```python
from build123d import *

# Parameters (mm, degrees)
BOSS_EXTRUDE1_DEPTH      = 1
SKETCH2_W                = 9
SKETCH2_H                = 4
BOSS_EXTRUDE2_DEPTH      = 1.5
BOSS_EXTRUDE5_DEPTH      = 8
BOSS_EXTRUDE5_DEPTH_BACK = 8


with BuildPart() as part:
    # Sketch1 → Boss-Extrude1 (new body)
    with BuildSketch(Plane.XY):
        Polygon((-63, -10), (-70, -10), (-70, 10), (-63, 10), (-63, 30.8), (-110.8, 30.8), (-110.8, -30.8), (-63, -30.8), align=None)
    extrude(amount=-BOSS_EXTRUDE1_DEPTH)

    # Sketch2 → Boss-Extrude2 (add)
    with BuildSketch(Plane(origin=(0, 0, -1), x_dir=(-1, 0, 0), z_dir=(0, 0, -1))):
        with Locations((110.8, -10)):
            Rectangle(SKETCH2_W, SKETCH2_H)
        with Locations((110.8, 10)):
            Rectangle(SKETCH2_W, SKETCH2_H)
    extrude(amount=BOSS_EXTRUDE2_DEPTH)

    # Sketch4 → Boss-Extrude5 (add, two sides: drawn at the far end of the back side and taken through both)
    with BuildSketch(Plane(origin=(0, 0, 0), x_dir=(1, 0, 0), z_dir=(0, 1, 0)).offset(-BOSS_EXTRUDE5_DEPTH_BACK)):
        with BuildLine():
            Line((-63.746646239, 13.303022537), (-63.062370045, 2))
            Line((-63.062370045, 2), (-64.5, 2))
            Line((-64.5, 2), (-64.5, -0.2))
            Line((-64.5, -0.2), (-63.5, -0.2))
            Line((-63.5, -0.2), (-63.5, 1))
            Line((-63.5, 1), (-62, 1))
            Line((-62, 1), (-62.790668189, 14.060428588))
            ThreePointArc((-62.790668189, 14.060428588), (-63.7786518, 14.999948092), (-64.785574648, 14.080755571))
            Line((-64.785574648, 14.080755571), (-65.688532626, 2.935903953))
            ThreePointArc((-65.688532626, 2.935903953), (-66.359873651, 1.557863976), (-67.787627389, 1))
            Line((-67.787627389, 1), (-70, 1))
            Line((-70, 1), (-70, 0))
            Line((-70, 0), (-67.787627389, 0))
            ThreePointArc((-67.787627389, 0), (-65.681919218, 0.822760048), (-64.691798691, 2.855148382))
            Line((-64.691798691, 2.855148382), (-63.845228573, 13.304027036))
            ThreePointArc((-63.845228573, 13.304027036), (-63.795469446, 13.349450792), (-63.746646239, 13.303022537))
        make_face()
    extrude(amount=BOSS_EXTRUDE5_DEPTH + BOSS_EXTRUDE5_DEPTH_BACK)


solid = part.part
```
Read the model definition and answer for the solid it produces. Units are mm, in the model's axes. A direction names the side the tool comes from. Round coordinates to 2 decimals unless told otherwise and drop trailing zeros. Write each loop counter-clockwise with the first axis right and the second up, starting at its lowest first coordinate (ties: lowest second). Pieces come first, ordered by that corner, then holes. Notation, with made-up numbers: (-32.5, -20) - (7.5, -20) arc R9 cw to (7.5, -12) - close; hole circle Ø1 at (3.25, 77). An arc over 180 degrees is marked (long way). One line per item, written item: value.
Q1. Find section A-A (y = 2). Determine the outline of the cut face in (x, z), and give its area (3 significant figures).
The answers:
outline: (-110.8, -1) - (-67.79, -1) arc R2.11 cw to (-65.69, -2.94) - (-64.79, -14.08) arc R1 ccw to (-62.79, -14.06) - (-62, -1) - (-63.5, -1) - (-63.5, 0.2) - (-64.5, 0.2) - (-64.5, -2) - (-63.06, -2) - (-63.75, -13.3) arc R0.05 cw to (-63.85, -13.3) - (-64.69, -2.86) arc R3.11 ccw to (-67.79, 0) - (-110.8, 0) - close
area: 75.3 mm2
Q2. Find section D-D (y = -21). Determine the outline of the cut face in (x, z).
The answers:
outline: (-110.8, -1) - (-63, -1) - (-63, 0) - (-110.8, 0) - close
Q3. Find section C-C (x = -103). Determine the outline of the cut face in (y, z), and give its area (3 significant figures).
The answers:
outline: (-30.8, -1) - (30.8, -1) - (30.8, 0) - (-30.8, 0) - close
area: 61.6 mm2
Q4. Straight lines are drawn through the part: line 1 (Y direction, x = -109, z = -1.5); line 2 (Z direction, x = -87.5, y = -19); line 3 (Z direction, x = -112, y = -9). For each, find the intervals that lie inside material, in ascending order. Write a range as from..to.
The answers:
line 1: y = -12..-8, 8..12
line 2: z = -1..0
line 3: z = -2.5..-1
Q5. Which of the six approach directions +Z, -Z, +X, -X, +Y, -Y give full straight-line access (tool end or side, diameter ignored) to faces 5 (the flat face through (-65, -8, -6)), 6 (the flat face through (-113, 10, -1)), 7 (the flat face through (-115.3, 10, -2)), 8 (the flat face through (-106.3, -10, -2)), 9 (the flat face through (-64.274, -0.112, -8.006))?
The answers:
face 5: +Z, -Z, +X
face 6: +Z, -X, +Y, -Y
face 7: +Z, -Z, -X, +Y, -Y
face 8: -Z, +X, +Y, -Y
face 9: +Y, -Y
Q6. Find section B-B (z = -12). Determine the outline of the cut face in (x, y).
The answers:
outline: (-64.95, -8) - (-63.95, -8) - (-63.95, 8) - (-64.95, 8) - close; (-63.67, -8) - (-62.67, -8) - (-62.67, 8) - (-63.67, 8) - close
Q7. For a pull along Y with two mould halves and no side action, classify faces 1 (the flat face through (-111, 12, -2)), 2 (the flat face through (-64, 0, -2)), 3 (the flat face through (-111, 8, -2)), 4 (the flat face through (-111, -12, -2)) as pulls with the +Y half, pulls with the -Y half, needs draft (parallel to the pull), parting line crosses it, or undercut.
The answers:
face 1: pulls with the +Y half
face 2: needs draft
face 3: undercut
face 4: pulls with the -Y half
Q8. Each of these flat-tipped pins is pushed along its axis until it touches: P1, Ø4, axis at x = -67, z = -7, coming from the +Y side; P2, Ø4, axis at x = -109.5, z = -3.5, coming from the -Y side; P3, Ø1, axis at y = -0.5, z = 0, coming from the +X side; P4, Ø6, axis at x = -68.5, z = -12.5, coming from the +Y side. Where does it stop, or does it pass through?
The answers:
P1: stops at y = 8
P2: stops at y = -12
P3: stops at x = -63.5
P4: passes through
